Autodesk Inventor part; units mm, degrees
ref_plane "YZ Plane" through (0, 0, 0) normal (1, 0, 0) x (0, 1, 0)
ref_plane "XZ Plane" through (0, 0, 0) normal (0, 1, 0) x (-1, 0, 0)
ref_plane "XY Plane" through (0, 0, 0) normal (0, 0, 1) x (1, 0, 0)
sketch "Эскиз1" plane through (0, 0, 0) normal (0, 0, 1) x (1, 0, 0)
  line L0 (-35, 15) -> (35, 15)
  line L1 (35, 15) -> (35, -15)
  line L2 (35, -15) -> (-35, -15)
  line L3 (-35, -15) -> (-35, 15)
  point P0 (0, 0)
  dimension "d0" = 70
  dimension "d1" = 30
  dimension "d2" = 15
  dimension "d3" = 35
extrude "Выдавливание1" add sketch "Эскиз1" along normal blind 12
sketch "Эскиз2" plane through (0, 0, 12) normal (0, 0, 1) x (1, 0, 0)
  line L0 (-35, 6) -> (-23, 6)
  line L1 (-23, 6) -> (-23, -6)
  line L2 (-23, -6) -> (-35, -6)
  line L3 (-35, -6) -> (-35, 6)
  point P0 (0, 0)
  dimension "d6" = 6
  dimension "d7" = 6
  dimension "d8" = 12
  dimension "d9" = 35
extrude "Выдавливание2" cut sketch "Эскиз2" against normal blind 12
sketch "Эскиз3" plane through (-35, -15, 0) normal (0, -1, 0) x (1, 0, 0)
  line L0 (70, 0) -> (0, 0)
  line L1 (20, 0) -> (50, 0)
  line L2 (50, 0) -> (50, 5)
  line L3 (50, 5) -> (20, 5)
  line L4 (20, 5) -> (20, 0)
  point P0 (35, 0)
  dimension "d12" = 30
  dimension "d13" = 5
  dimension "d14" = 20
extrude "Выдавливание3" cut sketch "Эскиз3" against normal blind 30
sketch "Эскиз4" plane through (0, 0, 12) normal (0, 0, 1) x (1, 0, 0)
  line L0 (-10, 15) -> (15, 15)
  line L1 (15, 15) -> (15, 7)
  line L2 (15, 7) -> (-10, 7)
  line L3 (-10, 7) -> (-10, 15)
  line L4 (15, -15) -> (-10, -15)
  line L5 (-10, -15) -> (-10, -7)
  line L6 (-10, -7) -> (15, -7)
  line L7 (15, -7) -> (15, -15)
  line L8 (35, -15) -> (35, 15)
  line L9 (-35, 15) -> (-35, 6)
  line L10 (-35, -6) -> (-35, -15)
  line L11 (-35, 6) -> (-23, 6)
  line L12 (-23, 6) -> (-23, -6)
  line L13 (-23, -6) -> (-35, -6)
  line L14 (-35, -6) -> (-35, -15)
  line L15 (-35, -15) -> (35, -15)
  line L16 (35, -15) -> (35, 15)
  line L17 (35, 15) -> (-35, 15)
  line L18 (-35, 15) -> (-35, 6)
  point P0 (0, 0)
  dimension "d17" = 20
  dimension "d18" = 20
  dimension "d19" = 25
  dimension "d20" = 25
  dimension "d21" = 14
  dimension "d22" = 8
  dimension "d23" = 8
  dimension "d24" = 7
extrude "Выдавливание4" add sketch "Эскиз4" along normal blind 6 contours L0 L1 L2 L3 | L4 L5 L6 L7
sketch "Эскиз5" plane through (0, 0, 12) normal (0, 0, 1) x (1, 0, 0)
  line L0 (15, 15) -> (35, 15)
  line L1 (35, 15) -> (35, -15)
  line L2 (35, -15) -> (15, -15)
  line L3 (15, -15) -> (15, 15)
  point P0 (0, 0)
extrude "Выдавливание5" add sketch "Эскиз5" along normal blind 18
sketch "Эскиз6" plane through (15, -7, 12) normal (-1, 0, 0) x (0, 0, 1)
  circle A0 centre (18, 7) radius 15
  point P0 (-12, 7)
  point P1 (18, 22)
  point P2 (18, -8)
  dimension "d29" = 30
extrude "Выдавливание6" add sketch "Эскиз6" against normal blind 20
sketch "Эскиз7" plane through (15, -7, 12) normal (-1, 0, 0) x (0, 0, 1)
  line L0 (0, 14) -> (6, 14)
  line L1 (0, 0) -> (0, 14)
  line L2 (0, 0) -> (6, 0)
  line L3 (6, -8) -> (6, 0)
  line L4 (6, -8) -> (18, -8)
  arc A0 (18, -8) -> (18, 22) centre (18, 7) ccw
  line L5 (6, 22) -> (18, 22)
  line L6 (6, 14) -> (6, 22)
  point P0 (-12, 7)
hole "Отверстие1" at (15, 0, 30) direction (1, 0, 0) diameter 20 depth 20 tip angle 118
properties part number "трон"
For this review, take the finished solid that the model builds, in its own axes (mm). A direction names the side the tool comes from. Give positions to 0.01 mm unless a question says otherwise; leave off trailing zeros. Write each loop counter-clockwise with the first axis right and the second up, starting at its lowest first coordinate (ties: lowest second). Pieces come first, ordered by that corner, then holes.
Item 1: Take a section at D-D (x = -13). Give the boundary of the cut face in (y, z), and give its area (3 significant figures).
Item 2: The part is to be moulded in two halves that separate along Y. For faces 6 (the face through (8, -15, 11)), 7 (the face through (-10, 0, 12)), 8 (the face through (25, 0, 0)), say which applies: +Y half, -Y half, draft (parallel to the pull), parting line (faces both ways), or undercut.
Item 3: Wall thickness on probe 1 along Z at (x, y) = (23.5, 0); probe 2 along Y at (x, z) = (28, 30); probe 3 along Y at (x, z) = (14.5, 16.5): over which ranges is each line inside the solid? List them lowest first.
Item 4: Take a section at B-B (z = 3). Give the boundary of the cut face in (x, y), and give its area (3 significant figures).
Item 5: Take a section at C-C (z = 14). Give the boundary of the cut face in (x, y), and give its area (3 significant figures).
Item 6: Insertion check: P1, Ø5, axis at x = -13.5, y = 11.5, coming from the +Z side; P2, Ø6.5, axis at y = 10.5, z = 16.5, coming from the -X side; P3, Ø3, axis at x = -8, y = -7, coming from the +Z side. Each pin has a flat end and moves straight along its axis. Give the tip position at first contact, or say it passes through.
Item 7: Take a section at A-A (y = 0). Give the boundary of the cut face in (x, z).
Item 8: Machinability: for faces 1 (the face through (2, -7, 15)), 2 (the face through (0, 0, 5)), 3 (the face through (-21, 0, 0)), 4 (the face through (-29, 6, 6)), 5 (the face through (-10, 11, 15)), which of the approach directions +Z, -Z, +X, -X, +Y, -Y give a long, thin tool a straight path to every point of the face, cutting with its end or side? Answer none if there is none.
Established:
1. outline: (-15, 5) - (15, 5) - (15, 12) - (-15, 12) - close
1. area: 210 mm2
2. face 6: -Y half
2. face 7: undercut
2. face 8: draft
3. probe 1: z = 0 to 20, 40 to 45
3. probe 2: y = -15 to -10, 10 to 15
3. probe 3: y = -15 to -7, 7 to 15
4. outline: (-35, -15) - (-15, -15) - (-15, 15) - (-35, 15) - (-35, 6) - (-23, 6) - (-23, -6) - (-35, -6) - close; (15, -15) - (35, -15) - (35, 15) - (15, 15) - close
4. area: 1,060 mm2
5. outline: (-10, -15) - (35, -15) - (35, 15) - (-10, 15) - (-10, 7) - (15, 7) - (15, -7) - (-10, -7) - close
5. area: 1,000 mm2
6. P1: stops at z = 12
6. P2: stops at x = -10
6. P3: stops at z = 18
7. outline: (-23, 0) - (-15, 0) - (-15, 5) - (15, 5) - (15, 0) - (35, 0) - (35, 20) - (15, 20) - (15, 12) - (-23, 12) - close; (15, 40) - (35, 40) - (35, 45) - (15, 45) - close
8. face 1: +Z, -X
8. face 2: -Z, +Y, -Y
8. face 3: -Z, +X, -X, +Y, -Y
8. face 4: +Z, -Z, -X
8. face 5: +Z, -X, +Y, -Y
